from build123d import *

# Parameters (mm, degrees)
BOSS_EXTRUDE1_DEPTH = 12.7


with BuildPart() as part:
    # Sketch1 → Boss-Extrude1 (new body)
    with BuildSketch(Plane(origin=(0, 0, 0), x_dir=(1, 0, 0), z_dir=(0, 1, 0))):
        with BuildLine():
            Line((-188.341, 198.501), (188.341, 198.501))
            ThreePointArc((188.341, 198.501), (195.525204897, 195.525204897), (198.501, 188.341))
            Line((198.501, 188.341), (198.501, -188.341))
            ThreePointArc((198.501, -188.341), (195.525204897, -195.525204897), (188.341, -198.501))
            Line((188.341, -198.501), (-188.341, -198.501))
            ThreePointArc((-188.341, -198.501), (-195.525204897, -195.525204897), (-198.501, -188.341))
            Line((-198.501, -188.341), (-198.501, 188.341))
            ThreePointArc((-198.501, 188.341), (-195.525204897, 195.525204897), (-188.341, 198.501))
        make_face()
        with BuildLine():
            Line((-170.4975, 173.0375), (-170.4975, 162.8775))
            ThreePointArc((-170.4975, 162.8775), (-173.0375, 160.3375), (-175.5775, 162.8775))
            Line((-175.5775, 162.8775), (-175.5775, 173.0375))
            ThreePointArc((-175.5775, 173.0375), (-173.0375, 175.5775), (-170.4975, 173.0375))
        make_face(mode=Mode.SUBTRACT)
        with BuildLine():
            Line((175.5775, 173.0375), (175.5775, 162.8775))
            ThreePointArc((175.5775, 162.8775), (173.0375, 160.3375), (170.4975, 162.8775))
            Line((170.4975, 162.8775), (170.4975, 173.0375))
            ThreePointArc((170.4975, 173.0375), (173.0375, 175.5775), (175.5775, 173.0375))
        make_face(mode=Mode.SUBTRACT)
        with BuildLine():
            Line((-170.4975, -173.0375), (-170.4975, -183.1975))
            ThreePointArc((-170.4975, -183.1975), (-173.0375, -185.7375), (-175.5775, -183.1975))
            Line((-175.5775, -183.1975), (-175.5775, -173.0375))
            ThreePointArc((-175.5775, -173.0375), (-173.0375, -170.4975), (-170.4975, -173.0375))
        make_face(mode=Mode.SUBTRACT)
        with BuildLine():
            Line((175.5775, -173.0375), (175.5775, -183.1975))
            ThreePointArc((175.5775, -183.1975), (173.0375, -185.7375), (170.4975, -183.1975))
            Line((170.4975, -183.1975), (170.4975, -173.0375))
            ThreePointArc((170.4975, -173.0375), (173.0375, -170.4975), (175.5775, -173.0375))
        make_face(mode=Mode.SUBTRACT)
    extrude(amount=BOSS_EXTRUDE1_DEPTH)


solid = part.part
CAD build for the part. Positions are in the model's coordinates, mm. A direction names the side the tool comes from. Give positions to 0.01 mm unless a question says otherwise; leave off trailing zeros. One line per question, with ' | ' between items. Start each with the question number.
1. Probe L1, parallel to X at y = 5.5, z = -165; L2, parallel to X at y = 9.5, z = -174. List the from-to ranges inside material, lowest first. Write a range as from..to.
2. 3-axis set-ups, long thin cutter, end or side, ignore diameter. For faces 1 (the face through (170.498, 6, 178)), 2 (the face through (-195.6, 6.26, -195.45)): which of +Z, -Z, +X, -X, +Y, -Y reach the whole face in a straight line?
3. Two-plate mould, pull along Z, no slides. Class faces 3 (the face through (175.578, 6, 178)), 4 (the face through (195.45, 6.26, -195.6)), 5 (the face through (195.6, 6.26, 195.45)): pulls with the +Z half, pulls with the -Z half, needs draft (parallel to the pull), parting line crosses it, or undercut.
Result sheet:
1) L1: x = -198.5..-175.58, -170.5..170.5, 175.58..198.5 | L2: x = -198.5..-175.39, -170.69..170.69, 175.39..198.5
2) face 1: +Y, -Y | face 2: -Z, -X, +Y, -Y
3) face 3: undercut | face 4: pulls with the -Z half | face 5: pulls with the +Z half
